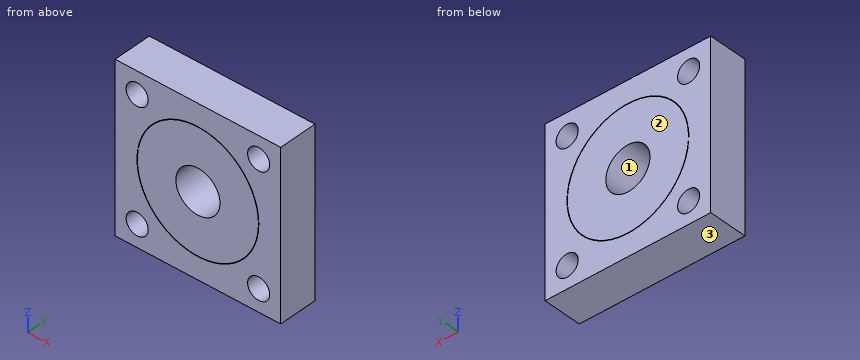
```python
from build123d import *

# Parameters (mm, degrees)
SKETCH1_W                    = 30
SKETCH1_H                    = 30
SKETCH1_R                    = 4
BOSS_EXTRUDE1_DEPTH          = 7
CUT_EXTRUDE_THIN1_DEPTH      = 1
CUT_EXTRUDE_THIN1_DEPTH_BACK = 10
SKETCH3_R                    = 2
CUT_EXTRUDE1_DEPTH           = 10
CIRPATTERN1_COUNT            = 4


with BuildPart() as part:
    # Sketch1 → Boss-Extrude1 (new body)
    with BuildSketch(Plane(origin=(0, 0, 0), x_dir=(1, 0, 0), z_dir=(0, 1, 0))):
        Rectangle(SKETCH1_W, SKETCH1_H)
        Circle(SKETCH1_R, mode=Mode.SUBTRACT)
    extrude(amount=BOSS_EXTRUDE1_DEPTH)

    # Sketch2 → Cut-Extrude-Thin1 (cut, two sides)
    with BuildSketch(Plane.XZ) as cut_extrude_thin1_sk:
        with BuildLine():
            ThreePointArc((-10.891369385, 1.805456431), (10.875199295, -1.900431606), (-10.858201017, 1.995262057))
            Line((-10.858201017, 1.995262057), (-10.779518401, 1.980803636))
            ThreePointArc((-10.779518401, 1.980803636), (10.796393503, -1.886660363), (-10.812446418, 1.792373414))
            Line((-10.812446418, 1.792373414), (-10.891369385, 1.805456431))
        make_face()
    extrude(amount=CUT_EXTRUDE_THIN1_DEPTH, mode=Mode.SUBTRACT)
    extrude(cut_extrude_thin1_sk.sketch, amount=-CUT_EXTRUDE_THIN1_DEPTH_BACK, mode=Mode.SUBTRACT)

    # Sketch3 → Cut-Extrude1 (cut)
    with BuildSketch(Plane(origin=(0, 7, 0), x_dir=(1, 0, 0), z_dir=(0, 1, 0))):
        with Locations((11, 11)):
            Circle(SKETCH3_R)
    cut_extrude1 = extrude(amount=-CUT_EXTRUDE1_DEPTH, mode=Mode.SUBTRACT)

    # CirPattern1: Cut-Extrude1 ×4 about axis
    cirpattern1_axis = Axis((0, 0, 0), (0, 1, 0))
    for i in range(1, CIRPATTERN1_COUNT):
        add(cut_extrude1.rotate(cirpattern1_axis, i * 360 / CIRPATTERN1_COUNT), mode=Mode.SUBTRACT)


solid = part.part
```
Verification items for the finished model (mm, model axes). Face numbers are marked on the shaded views. Round coordinates to 2 decimals unless told otherwise and drop trailing zeros. Order: outer loops, then holes, each group sorted by start corner. A loop starts at its lowest first (then second) coordinate and runs counter-clockwise, first axis right, second up.
1) Cross-section at C-C, the plane x = 1.5. Record the cut outline in (y, z).
Geometry says:
outline: (0, -15) - (7, -15) - (7, -10.94) - (0, -10.94) - close; (0, -10.86) - (7, -10.86) - (7, -3.71) - (0, -3.71) - close; (0, 3.71) - (7, 3.71) - (7, 10.86) - (0, 10.86) - close; (0, 10.94) - (7, 10.94) - (7, 15) - (0, 15) - close
2) Material ranges on line 1 (Z direction, x = 11.5, y = 3.75); line 2 (X direction, y = 6.5, z = 9.5), recorded low to high.
Geometry says:
line 1: z = -15 to -12.94, -9.06 to 9.06, 12.94 to 15
line 2: x = -15 to -12.32, -9.68 to -5.62, -5.47 to 5.47, 5.62 to 9.68, 12.32 to 15
3) Cross-section at D-D, the plane z = 9.75. Record the cut outline in (x, y).
Geometry says:
outline: (-15, 0) - (-12.56, 0) - (-12.56, 7) - (-15, 7) - close; (-9.44, 0) - (-5.18, 0) - (-5.18, 7) - (-9.44, 7) - close; (-5.01, 0) - (5.01, 0) - (5.01, 7) - (-5.01, 7) - close; (5.18, 0) - (9.44, 0) - (9.44, 7) - (5.18, 7) - close; (12.56, 0) - (15, 0) - (15, 7) - (12.56, 7) - close
4) Cross-section at B-B, the plane z = 0. Record the cut outline in (x, y), plus the area to 3 significant figures.
Geometry says:
outline: (-15, 0) - (-11.04, 0) - (-11.04, 7) - (-15, 7) - close; (-10.96, 0) - (-4, 0) - (-4, 7) - (-10.96, 7) - close; (4, 0) - (10.96, 0) - (10.96, 7) - (4, 7) - close; (11.04, 0) - (15, 0) - (15, 7) - (11.04, 7) - close
area: 153 mm2
5) Draft check along Z on the marked faces 1, 2 and 3. Enter one of: +Z half, -Z half, draft (parallel to the pull), parting line (faces both ways), or undercut.
Geometry says:
face 1: undercut
face 2: draft
face 3: -Z half
6) Depth check by flat-ended pin: pin 1 (2.5 mm diameter, centred on x = 11, z = 11, fed in from +Y). Enter the tip coordinate at first touch or a pass-through.
Geometry says:
pin 1: passes through
7) Cross-section at A-A, the plane y = 4. Record the cut outline in (x, z).
Geometry says:
outline: (-15, -15) - (15, -15) - (15, 15) - (-15, 15) - close; hole circle Ø4 at (-11, -11); hole circle Ø4 at (-11, 11); hole (-10.89, 1.81) arc R11.04 ccw (long way) to (-10.86, 2) - (-10.78, 1.98) arc R10.96 cw (long way) to (-10.81, 1.79) - close; hole circle Ø8 at (0, 0); hole circle Ø4 at (11, -11); hole circle Ø4 at (11, 11)
